from build123d import *

# Parameters (mm, degrees)
SKETCH_R   = 15
SKETCH_R_2 = 3
PAD_DEPTH  = 10
FILLET_R   = 3


with BuildPart() as part:
    # Sketch → Pad (new body)
    with BuildSketch(Plane.XY):
        with BuildLine():
            Line((0, 12.5), (200, 12.5))
            Line((200, 12.5), (200, 187.5))
            Line((200, 187.5), (0, 187.5))
            Line((0, 187.5), (0, 166.424769))
            ThreePointArc((0, 33.575231), (55.5, 100), (0, 166.424769))
            Line((0, 12.5), (0, 33.575231))
        make_face()
        with Locations((136, 100)):
            Circle(SKETCH_R, mode=Mode.SUBTRACT)
        with Locations((118.32233, 117.67767)):
            Circle(SKETCH_R_2, mode=Mode.SUBTRACT)
        with Locations((153.67767, 117.67767)):
            Circle(SKETCH_R_2, mode=Mode.SUBTRACT)
        with Locations((118.32233, 82.32233)):
            Circle(SKETCH_R_2, mode=Mode.SUBTRACT)
        with Locations((153.67767, 82.32233)):
            Circle(SKETCH_R_2, mode=Mode.SUBTRACT)
        with Locations((40, 25.5)):
            Circle(SKETCH_R_2, mode=Mode.SUBTRACT)
        with Locations((160, 25.5)):
            Circle(SKETCH_R_2, mode=Mode.SUBTRACT)
        with Locations((80, 25.5)):
            Circle(SKETCH_R_2, mode=Mode.SUBTRACT)
        with Locations((120, 25.5)):
            Circle(SKETCH_R_2, mode=Mode.SUBTRACT)
        with Locations((40, 174.5)):
            Circle(SKETCH_R_2, mode=Mode.SUBTRACT)
        with Locations((80, 174.5)):
            Circle(SKETCH_R_2, mode=Mode.SUBTRACT)
        with Locations((120, 174.5)):
            Circle(SKETCH_R_2, mode=Mode.SUBTRACT)
        with Locations((160, 174.5)):
            Circle(SKETCH_R_2, mode=Mode.SUBTRACT)
        with Locations((187, 149.5)):
            Circle(SKETCH_R_2, mode=Mode.SUBTRACT)
        with Locations((187, 116.5)):
            Circle(SKETCH_R_2, mode=Mode.SUBTRACT)
        with Locations((187, 83.5)):
            Circle(SKETCH_R_2, mode=Mode.SUBTRACT)
        with Locations((187, 50.5)):
            Circle(SKETCH_R_2, mode=Mode.SUBTRACT)
    extrude(amount=PAD_DEPTH)

    # Fillet
    fillet_edges = [part.edges().sort_by_distance(p)[0] for p in [
        (0, 12.5, 5),
        (0, 33.575231, 5),
        (0, 166.424769, 5),
        (0, 187.5, 5),
        (200, 12.5, 5),
        (200, 187.5, 5),
    ]]
    fillet(fillet_edges, radius=FILLET_R)


solid = part.part
The listing builds one solid part. Answer for the finished solid, in the listing's coordinates (mm). Coordinates: 2 decimals unless noted, no trailing zeros. Loops run counter-clockwise (first coordinate to the right, second up) from the corner with the lowest first, then second, coordinate; pieces in that order, holes last. Notation, with made-up numbers: (-25, 71) -> (-8, 71) arc R33 ccw to (-8, 100) -> close; hole circle Ø7 at (63.25, 5). An arc over 180 degrees is marked (long way). Write item = value, one per line. Start each with the question number.
1) A cutting plane is placed at C-C (x = 160). Give the vertices of the cut face in (y, z).
2) A cutting plane is placed at A-A (y = 25.5). Give the vertices of the cut face in (x, z), then the cut area to 3 significant figures.
3) The mould has two halves that part along Y. Classify faces 1 (the face through (99, 12.5, 5)), 2 (the face through (120.8, 101.2, 10)), 3 (the face through (121.61, 177.03, 4.93)): released by +Y, released by -Y, zero draft, split by the parting line, or undercut.
4) A cutting plane is placed at D-D (z = 2.25). Count the separate pieces of the cut face and the enclosed holes in it, then the cut area to 3 significant figures.
5) Given pin 1 Ø3.5 at (x, y) = (120, 174.5) entering from +Z; pin 2 Ø5 at (y, z) = (126.5, 6) entering from -X, each flat-ended and moving along its own axis, determine where each tip first touches the part or whether it passes through.
6) A cutting plane is placed at B-B (y = 100). Give the vertices of the cut face in (x, z).
7) Straight lines are drawn through the part: line 1 (Y direction, x = 187, z = 5); line 2 (X direction, y = 174.5, z = 1.25); line 3 (Y direction, x = 120, z = 6). For each, find the intervals that lie inside material, in ascending order. Write a range as from..to.
Responses:
q1.outline = (12.5, 0) -> (22.5, 0) -> (22.5, 10) -> (12.5, 10) -> close; (28.5, 0) -> (171.5, 0) -> (171.5, 10) -> (28.5, 10) -> close; (177.5, 0) -> (187.5, 0) -> (187.5, 10) -> (177.5, 10) -> close
q2.outline = (0, 0) -> (37, 0) -> (37, 10) -> (0, 10) -> close; (43, 0) -> (77, 0) -> (77, 10) -> (43, 10) -> close; (83, 0) -> (117, 0) -> (117, 10) -> (83, 10) -> close; (123, 0) -> (157, 0) -> (157, 10) -> (123, 10) -> close; (163, 0) -> (200, 0) -> (200, 10) -> (163, 10) -> close
q2.area = 1,760 mm²
q3.face_1 = released by -Y
q3.face_2 = zero draft
q3.face_3 = undercut
q4.separate_pieces = 1
q4.enclosed_holes = 17
q4.area = 28,300 mm²
q5.pin_1 = through
q5.pin_2 = 48.95
q6.outline = (55.5, 0) -> (121, 0) -> (121, 10) -> (55.5, 10) -> close; (151, 0) -> (200, 0) -> (200, 10) -> (151, 10) -> close
q7.line_1 = 12.5..47.5, 53.5..80.5, 86.5..113.5, 119.5..146.5, 152.5..187.5
q7.line_2 = 0..37, 43..77, 83..117, 123..157, 163..200
q7.line_3 = 12.5..22.5, 28.5..79.84, 84.81..115.19, 120.16..171.5, 177.5..187.5
